Could you check a few things on this model? Use its own coordinates, in mm. Coordinates: 2 decimals unless noted, no trailing zeros. Loops run counter-clockwise (first coordinate to the right, second up) from the corner with the lowest first, then second, coordinate; pieces in that order, holes last. Notation, with made-up numbers: (23.5, 47) -> (48.5, 47) arc R26 cw to (48.5, 75) -> close; hole circle Ø7 at (-20, -31.5). An arc over 180 degrees is marked (long way). One line per question, with ' | ' between items.
from build123d import *

# Parameters (mm, degrees)
SKETCH_1_R      = 2.6
SKETCH_1_W      = 15
SKETCH_1_H      = 15
EXTRUDE_1_DEPTH = 2


with BuildPart() as part:
    # 草图1 → 凸台-拉伸1 (new body)
    # profile 1 of 2: a face of its own
    with BuildSketch(Plane(origin=(0, 0, 0), x_dir=(1, 0, 0), z_dir=(0, 1, 0))):
        Polygon((7.5, -15), (7.5, 0), (7.5, 13), (7.5, 28), (-7.5, 28), (-7.5, 13), (-7.5, 0), (-22.5, 0), (-22.5, -15), align=None)
        with Locations(Location((-15, -7.5, 0), (0, 0, 270))):
            Circle(SKETCH_1_R, mode=Mode.SUBTRACT)
        with Locations(Location((0, -7.5, 0), (0, 0, 270))):
            Circle(SKETCH_1_R, mode=Mode.SUBTRACT)
        with Locations(Location((0, 20.5, 0), (0, 0, 270))):
            Circle(SKETCH_1_R, mode=Mode.SUBTRACT)
    # profile 2 of 2: a face of its own
    with BuildSketch(Plane(origin=(0, 0, 0), x_dir=(1, 0, 0), z_dir=(0, 1, 0))):
        with Locations((0, 35.5)):
            Rectangle(SKETCH_1_W, SKETCH_1_H)
        with Locations(Location((0, 35.5, 0), (0, 0, 270))):
            Circle(SKETCH_1_R, mode=Mode.SUBTRACT)
    extrude(amount=EXTRUDE_1_DEPTH)


solid = part.part
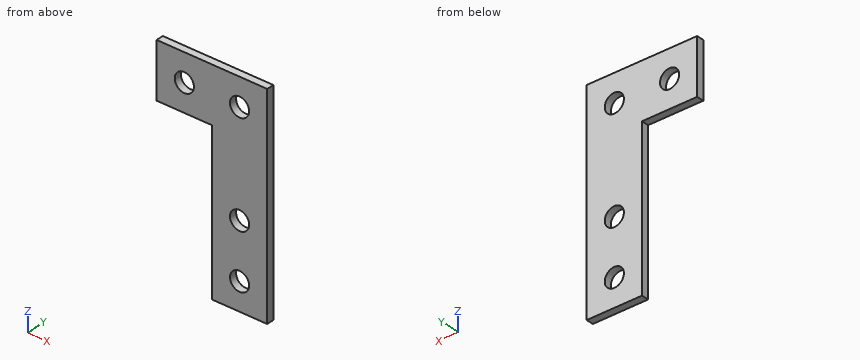
1) If we section it at D-D on z = 7.5: Please give me the cut outline in (x, y).
Data:
outline: (-22.5, 0) -> (-17.6, 0) -> (-17.6, 2) -> (-22.5, 2) -> close; (-12.4, 0) -> (-2.6, 0) -> (-2.6, 2) -> (-12.4, 2) -> close; (2.6, 0) -> (7.5, 0) -> (7.5, 2) -> (2.6, 2) -> close
2) I'm going to push flat-ended pins straight in: pin 1 Ø3 at (x, z) = (0, 7.5) entering from -Y; pin 2 Ø0.6 at (y, z) = (1, -17.5) entering from -X; pin 3 Ø7 at (x, z) = (-15, 7.5) entering from -Y; pin 4 Ø1 at (x, y) = (-12, 0.5) entering from -Z. Where does each tip first touch, or does it pass through?
Data:
pin 1: through | pin 2: x = -7.5 | pin 3: y = 0 | pin 4: z = 0
3) If we section it at C-C on x = -15: Please give me the cut outline in (y, z).
Data:
outline: (0, 0) -> (2, 0) -> (2, 4.9) -> (0, 4.9) -> close; (0, 10.1) -> (2, 10.1) -> (2, 15) -> (0, 15) -> close
4) I need wall thicknesses on line 1 along X through (y, z) = (1.2, 7.5); line 2 along X through (y, z) = (0.5, -35.5); line 3 along Z through (x, y) = (1, 0.7). Which ranges of each line are inside material? Lowest first, please. Write a range as from..to.
Data:
line 1: -22.5..-17.6, -12.4..-2.6, 2.6..7.5 | line 2: -7.5..-2.6, 2.6..7.5 | line 3: -43..-37.9, -33.1..-22.9, -18.1..5.1, 9.9..15
5) If we section it at A-A on z = -35.5: Please give me the cut outline in (x, y), and give its area (3 significant figures).
Data:
outline: (-7.5, 0) -> (-2.6, 0) -> (-2.6, 2) -> (-7.5, 2) -> close; (2.6, 0) -> (7.5, 0) -> (7.5, 2) -> (2.6, 2) -> close | area: 19.6 mm²
6) If we section it at B-B on y = 1.15: Please give me the cut outline in (x, z).
Data:
outline: (-22.5, 0) -> (-7.5, 0) -> (-7.5, -43) -> (7.5, -43) -> (7.5, 15) -> (-22.5, 15) -> close; hole circle Ø5.2 at (-15, 7.5); hole circle Ø5.2 at (0, -35.5); hole circle Ø5.2 at (0, -20.5); hole circle Ø5.2 at (0, 7.5)
